Model file for the job. Use its own axes, mm. A direction names the side the tool comes from. Coordinates: 2 decimals unless noted, no trailing zeros. Write each loop counter-clockwise with the first axis right and the second up, starting at its lowest first coordinate (ties: lowest second). Pieces come first, ordered by that corner, then holes.
Q1. Band-saw the part on B-B, the plane y = 8.25. Write the cut outline in (x, z).
Q2. Which spindle directions (+Z, -Z, +X, -X, +Y, -Y) get a long thin tool onto all of the face, cutting with end or side? Do faces 1 (the cylindrical face through (21.46, 7.22, -29.35)), 2 (the flat face through (-4, 4, 0)). Say none if no direction does.
Q3. Drill centre lines: probe 1 along Y at (x, z) = (22, -28); probe 2 along Y at (x, z) = (0, 2.5); probe 3 along X at (y, z) = (14.5, -25.5). Where is each one in solid material? Low to high.
Q4. Band-saw the part on C-C, the plane z = -19. Write the cut outline in (x, y), plus the area to 3 significant figures.
Q5. Band-saw the part on D-D, the plane x = 9. Write the cut outline in (y, z).
Q6. Pull direction X, two halves, no side cores. Call faces 3 (the cylindrical face through (-9.37, 6.59, 2.46)), 4 (the flat face through (19, 4, -15)), 5 (the flat face through (24, 0, -12)), 6 (the cylindrical face through (21.46, 1.5, -14.23)): released by +X, released by -X, zero draft, split by the parting line, or undercut.
Q7. Pin check, flat tips, straight feed: P1, Ø9, axis at y = 0, z = -19, coming from the +X side; P2, Ø5, axis at y = 1.5, z = -10, coming from the -X side; P3, Ø5.5, axis at x = -9, y = -8.25, coming from the -Z side. Stop position of each tip, or through.
Q8. Band-saw the part on A-A, the plane x = 0. Write the cut outline in (y, z).
from build123d import *

# Parameters (mm, degrees)
SKETCH1_W           = 38
SKETCH1_H           = 32
SKETCH1_R           = 5
SKETCH1_R_2         = 1.7
BOSS_EXTRUDE1_DEPTH = 5
SKETCH2_W           = 5
SKETCH2_H           = 32
BOSS_EXTRUDE4_DEPTH = 5


with BuildPart() as part:
    # Sketch1 → Boss-Extrude1 (new body)
    with BuildSketch(Plane.XY):
        Rectangle(SKETCH1_W, SKETCH1_H)
        Circle(SKETCH1_R, mode=Mode.SUBTRACT)
        with Locations((-9, 8.25)):
            Circle(SKETCH1_R_2, mode=Mode.SUBTRACT)
        with Locations((9, 8.25)):
            Circle(SKETCH1_R_2, mode=Mode.SUBTRACT)
        with Locations((9, -8.25)):
            Circle(SKETCH1_R_2, mode=Mode.SUBTRACT)
        with Locations((-9, -8.25)):
            Circle(SKETCH1_R_2, mode=Mode.SUBTRACT)
    boss_extrude1 = extrude(amount=BOSS_EXTRUDE1_DEPTH)

    # Sketch2 → Boss-Extrude4 (add)
    with BuildSketch(Plane.XY):
        with Locations((21.5, 0)):
            Rectangle(SKETCH2_W, SKETCH2_H)
    extrude(amount=BOSS_EXTRUDE4_DEPTH)

    # Mirror3: Boss-Extrude1 across plane
    add(boss_extrude1.mirror(Plane(origin=(9.5, 0, -9.5), x_dir=(0.7071067811865478, 0, 0.7071067811865472), z_dir=(0.7071067811865475, 0, -0.7071067811865477))))


solid = part.part
Answer sheet:
1. outline: (-19, 0) - (-10.7, 0) - (-10.7, 5) - (-19, 5) - close; (-7.3, 0) - (7.3, 0) - (7.3, 5) - (-7.3, 5) - close; (10.7, 0) - (19, 0) - (19, -8.3) - (24, -8.3) - (24, 5) - (10.7, 5) - close; (19, -38) - (24, -38) - (24, -29.7) - (19, -29.7) - close; (19, -26.3) - (24, -26.3) - (24, -11.7) - (19, -11.7) - close
2. face 1: +X, -X
2. face 2: -Z, -X, +Y, -Y
3. probe 1: y = -16 to -9.95, -6.55 to 6.55, 9.95 to 16
3. probe 2: y = -16 to -5, 5 to 16
3. probe 3: x = 19 to 24
4. outline: (19, -16) - (24, -16) - (24, -5) - (19, -5) - close; (19, 5) - (24, 5) - (24, 16) - (19, 16) - close
4. area: 110 mm2
5. outline: (-16, 0) - (-9.95, 0) - (-9.95, 5) - (-16, 5) - close; (-6.55, 0) - (6.55, 0) - (6.55, 5) - (-6.55, 5) - close; (9.95, 0) - (16, 0) - (16, 5) - (9.95, 5) - close
6. face 3: undercut
6. face 4: released by -X
6. face 5: released by +X
6. face 6: zero draft
7. P1: passes through
7. P2: stops at x = 19
7. P3: stops at z = 0
8. outline: (-16, 0) - (-5, 0) - (-5, 5) - (-16, 5) - close; (5, 0) - (16, 0) - (16, 5) - (5, 5) - close
